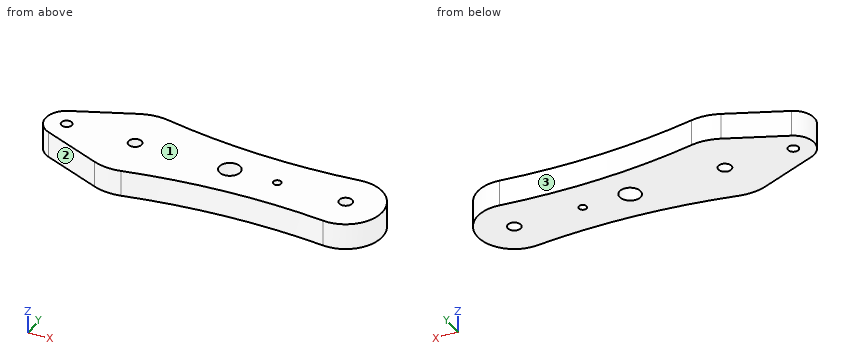
```python
from build123d import *

# Parameters (mm, degrees)
SKETCH1_R           = 1.25
SKETCH1_R_2         = 1
SKETCH1_R_3         = 2
SKETCH1_R_4         = 0.75
BOSS_EXTRUDE1_DEPTH = 5


with BuildPart() as part:
    # Sketch1 → Boss-Extrude1 (new body)
    with BuildSketch(Plane.XY):
        with BuildLine():
            Line((-14.538461538, 3.692307692), (-3.461538462, 8.307692308))
            ThreePointArc((-3.461538462, 8.307692308), (-0.847818166, 8.959977922), (1.841860465, 8.809514744))
            ThreePointArc((1.841860465, 8.809514744), (20.473513899, 6.416147504), (39.250393701, 6.959747869))
            ThreePointArc((39.250393701, 6.959747869), (47, 0), (39.250393701, -6.959747869))
            ThreePointArc((39.250393701, -6.959747869), (20.473513899, -6.416147504), (1.841860465, -8.809514744))
            ThreePointArc((1.841860465, -8.809514744), (-0.847818166, -8.959977922), (-3.461538462, -8.307692308))
            Line((-3.461538462, -8.307692308), (-14.538461538, -3.692307692))
            ThreePointArc((-14.538461538, -3.692307692), (-17, 0), (-14.538461538, 3.692307692))
        make_face()
        Circle(SKETCH1_R, mode=Mode.SUBTRACT)
        with Locations((40, 0)):
            Circle(SKETCH1_R, mode=Mode.SUBTRACT)
        with Locations((-13, 0)):
            Circle(SKETCH1_R_2, mode=Mode.SUBTRACT)
        with Locations((18, 0)):
            Circle(SKETCH1_R_3, mode=Mode.SUBTRACT)
        with Locations((27, 0)):
            Circle(SKETCH1_R_4, mode=Mode.SUBTRACT)
    extrude(amount=BOSS_EXTRUDE1_DEPTH)


solid = part.part
```
Geometry check sheet. Reference: the model listing, model coordinates, mm. Face numbers are marked on the shaded views. Give positions to 0.01 mm unless a question says otherwise; leave off trailing zeros. Write each loop counter-clockwise with the first axis right and the second up, starting at its lowest first coordinate (ties: lowest second). Pieces come first, ordered by that corner, then holes. Notation, with made-up numbers: (-18.5, 20) -> (-8.5, 20) arc R26 ccw to (-8.5, 45) -> close; hole circle Ø4 at (-33, 71). An arc over 180 degrees is marked (long way). One line per question, with ' | ' between items.
Item 1: Sectioned sample at B-B, the plane y = 0. Record the boundary of the cut face in (x, z).
Determined:
outline: (-17, 0) -> (-14, 0) -> (-14, 5) -> (-17, 5) -> close; (-12, 0) -> (-1.25, 0) -> (-1.25, 5) -> (-12, 5) -> close; (1.25, 0) -> (16, 0) -> (16, 5) -> (1.25, 5) -> close; (20, 0) -> (26.25, 0) -> (26.25, 5) -> (20, 5) -> close; (27.75, 0) -> (38.75, 0) -> (38.75, 5) -> (27.75, 5) -> close; (41.25, 0) -> (47, 0) -> (47, 5) -> (41.25, 5) -> close
Item 2: Draft check along X on the marked faces 1, 2 and 3. Enter one of: released by +X, released by -X, zero draft, split by the parting line, or undercut.
Determined:
face 1: zero draft | face 2: released by -X | face 3: undercut
Item 3: Sectioned sample at C-C, the plane z = 1.15. Record the boundary of the cut face in (x, y), plus the area to 3 significant figures.
Determined:
outline: (-14.54, -3.69) -> (-3.46, -8.31) arc R9 ccw to (1.84, -8.81) arc R120 cw to (39.25, -6.96) arc R7 ccw (long way) to (39.25, 6.96) arc R120 cw to (1.84, 8.81) arc R9 ccw to (-3.46, 8.31) -> (-14.54, 3.69) arc R4 ccw to start; hole circle Ø2 at (-13, 0); hole circle Ø2.5 at (0, 0); hole circle Ø4 at (18, 0); hole circle Ø1.5 at (27, 0); hole circle Ø2.5 at (40, 0) | area: 816 mm^2
Item 4: Sectioned sample at A-A, the plane x = 40. Record the boundary of the cut face in (y, z).
Determined:
outline: (-7, 0) -> (-1.25, 0) -> (-1.25, 5) -> (-7, 5) -> close; (1.25, 0) -> (7, 0) -> (7, 5) -> (1.25, 5) -> close
Item 5: Sectioned sample at D-D, the plane x = 27. Record the boundary of the cut face in (y, z).
Determined:
outline: (-6.27, 0) -> (-0.75, 0) -> (-0.75, 5) -> (-6.27, 5) -> close; (0.75, 0) -> (6.27, 0) -> (6.27, 5) -> (0.75, 5) -> close
Item 6: Scan lines: line 1 along X through (y, z) = (-0.5, 4.45); line 2 along X through (y, z) = (0.25, 3.7); line 3 along Y through (x, z) = (40, 3.05). Record each from-to range of solid material in increasing order.
Determined:
line 1: -16.97 to -13.87, -12.13 to -1.15, 1.15 to 16.06, 19.94 to 26.44, 27.56 to 38.85, 41.15 to 46.98 | line 2: -16.99 to -13.97, -12.03 to -1.22, 1.22 to 16.02, 19.98 to 26.29, 27.71 to 38.78, 41.22 to 47 | line 3: -7 to -1.25, 1.25 to 7
